Design review of the part built by this model. Coordinates are the model's own, in mm. Face numbers are marked on the shaded views. A direction names the side the tool comes from. Round coordinates to 2 decimals unless told otherwise and drop trailing zeros. Order: outer loops, then holes, each group sorted by start corner. A loop starts at its lowest first (then second) coordinate and runs counter-clockwise, first axis right, second up. Notation, with made-up numbers: M 56.25,-1.5 L 109.25,-1.5 A18 cw 109.25,25.5 Z; hole C 2,82.25 d10. An arc over 180 degrees is marked long. Use a Markdown table: item, result. Add a question column.
(1) Take a section at C-C (z = 0). Count the separate pieces of the cut face and the enclosed holes in it, then the cut area to 3 significant figures.
(2) For pin 1 (7 mm diameter, centred on y = 0, z = 0, fed in from +X); pin 2 (1.5 mm diameter, centred on x = -0.5, y = -9, fed in from -Z); pin 3 (2 mm diameter, centred on y = 8.5, z = 0, fed in from +X); pin 4 (3.5 mm diameter, centred on x = 0, z = 0, fed in from -Y), all flat-tipped, find the tip position at first contact; note any pin that passes through.
(3) Machinability: for the marked faces 1, 2 and 3, which of the approach directions +Z, -Z, +X, -X, +Y, -Y give a long, thin tool a straight path to every point of the face, cutting with its end or side? Answer none if there is none.
(4) The part is to be moulded in two halves that separate along Y. For the marked faces 4, 5 and 6, say which applies: released by +Y, released by -Y, zero draft, split by the parting line, or undercut.
(5) Take a section at A-A (x = 2.75). Write out the cut boundary in (y, z).
(6) To check wall thickness, follow probe 1 along Y at (x, z) = (0.25, 4); probe 2 along Y at (x, z) = (-6.75, 1); probe 3 along Y at (x, z) = (0, -1.5). State the ranges of each line that lie inside material, in increasing order. Write a range as from..to.
(7) Take a section at B-B (y = 0). Write out the cut boundary in (x, z).
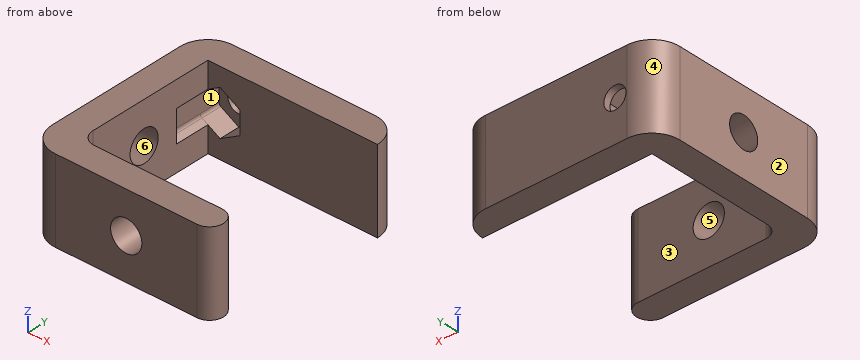
```python
from build123d import *

# Parameters (mm, degrees)
RESSALTO_EXTRUS_O1_DEPTH = 6
ESBO_O3_R                = 1.6
CORTE_EXTRUS_O1_DEPTH    = 4
CORTE_EXTRUS_O2_DEPTH    = 3
CORTE_EXTRUS_O3_DEPTH    = 5
FILETE1_R                = 0.5
FILETE2_R                = 4
FILETE3_R                = 2
ESBO_O6_R                = 2.25
CORTE_EXTRUS_O4_DEPTH    = 10
ESBO_O7_R                = 2.25
CORTE_EXTRUS_O5_DEPTH    = 10


# Some blends are built 0.0001 mm under size
with BuildPart() as part:
    # Esboço1 → Ressalto-extrusão1 (new, symmetric)
    with BuildSketch(Plane.XY):
        Polygon((14.2, 14.2), (-14.2, 14.2), (-14.2, -14.2), (14.2, -14.2), (14.2, -10.2), (10.2, -10.2), (-10.2, -10.2), (-10.2, 10.2), (10.2, 10.2), (14.2, 10.2), align=None)
    extrude(amount=RESSALTO_EXTRUS_O1_DEPTH, both=True)

    # Esboço3 → Corte-extrusão1 (cut)
    with BuildSketch(Plane(origin=(0, 14.2, 0), x_dir=(1, 0, 0), z_dir=(0, 1, 0))):
        with Locations(Location((-8.45, 0, 0), (0, 0, 270))):
            Circle(ESBO_O3_R)
    extrude(amount=-CORTE_EXTRUS_O1_DEPTH, mode=Mode.SUBTRACT)

    # Esboço4 → Corte-extrusão2 (cut)
    with BuildSketch(Plane.XZ.offset(-10.2)):
        Polygon((-8.45, 3.290896534), (-11.3, 1.645448267), (-11.3, -1.645448267), (-8.45, -3.290896534), (-5.6, -1.645448267), (-5.6, 1.645448267), align=None)
    extrude(amount=-CORTE_EXTRUS_O2_DEPTH, mode=Mode.SUBTRACT)

    # Esboço5 → Corte-extrusão3 (cut)
    with BuildSketch(Plane.XZ.offset(-10.2)):
        Polygon((-11.3, -1.645448267), (-10.2, -2.280533563), (-8.45, -3.290896534), (-5.6, -1.645448267), (-5.6, 1.645448267), (-8.45, 3.290896534), (-10.2, 2.280533563), (-11.3, 1.645448267), align=None)
    extrude(amount=CORTE_EXTRUS_O3_DEPTH, mode=Mode.SUBTRACT)

    # Filete1
    filete1_edges = [part.edges().sort_by_distance(p)[0] for p in [
        (-11.3, 9.2, -1.645448267),
        (-11.3, 9.2, 1.645448267),
        (-11.3, 5.2, 0),
    ]]
    fillet(filete1_edges, radius=FILETE1_R)

    # Filete2
    filete2_edges = [part.edges().sort_by_distance(p)[0] for p in [
        (-14.2, -14.2, 0),
        (-14.2, 14.2, 0),
        (14.2, 14.2, 0),
        (14.2, -14.2, 0),
    ]]
    fillet(filete2_edges, radius=FILETE2_R - 0.0001)  # a hair under: the kernel refuses the full size

    # Filete3
    # the kernel refuses this fillet: 2 mm, written as the material it adds along each edge
    with BuildSketch(Plane(origin=(-10.2, -10.2, -6), x_dir=(0, 1, 0), z_dir=(0, 0, 1))) as filete3_piece_1:
        with BuildLine():
            CenterArc((FILETE3_R, -FILETE3_R), FILETE3_R, 90, 90)
            Line((0, -FILETE3_R), (0, 0))
            Line((0, 0), (FILETE3_R, 0))
        make_face()
    extrude(amount=12)
    # the kernel refuses this fillet: 2 mm, written as the material it takes off along each edge
    with BuildSketch(Plane(origin=(14.2, -10.2, -20.141946005), x_dir=(-1, 0, 0), z_dir=(0, 0, 1))) as filete3_2_piece_1:
        with BuildLine():
            CenterArc((3.999896367, 2), FILETE3_R, 90.000104073, 179.999895927)
            Line((3.999892734, 4), (3.999892371, 4.2))
            ThreePointArc((3.999892371, 4.2), (-0.2, 0.0001), (-0.2, 0))
            Line((-0.2, 0), (0, -0.2))
            Line((0, -0.2), (3.999896367, -0.2))
            Line((3.999896367, -0.2), (3.999896367, 0))
        make_face()
    extrude(amount=40.283892009, mode=Mode.SUBTRACT)

    # Esboço6 → Corte-extrusão4 (cut)
    with BuildSketch(Plane.ZY.offset(14.2)):
        Circle(ESBO_O6_R)
    extrude(amount=-CORTE_EXTRUS_O4_DEPTH, mode=Mode.SUBTRACT)

    # Esboço7 → Corte-extrusão5 (cut)
    with BuildSketch(Plane.XZ.offset(14.2)):
        with Locations(Location((0, 0, 0), (0, 0, 270))):
            Circle(ESBO_O7_R)
    extrude(amount=-CORTE_EXTRUS_O5_DEPTH, mode=Mode.SUBTRACT)


solid = part.part
```
Verdict:
| question | item | result |
|---|---|---|
| 1 | separate pieces | 4 |
| 1 | enclosed holes | 0 |
| 1 | area | 228 mm^2 |
| 2 | pin 1 | stops at x = -10.2 |
| 2 | pin 2 | passes through |
| 2 | pin 3 | stops at x = -11.3 |
| 2 | pin 4 | stops at y = 10.2 |
| 3 | face 1 | none |
| 3 | face 2 | +Z, -Z, -X, +Y, -Y |
| 3 | face 3 | +Z, -Z, +X |
| 4 | face 4 | released by +Y |
| 4 | face 5 | zero draft |
| 4 | face 6 | undercut |
| 5 | outline | M -14.2,-6 L -10.2,-6 L -10.2,6 L -14.2,6 Z; M 10.2,-6 L 14.2,-6 L 14.2,6 L 10.2,6 Z |
| 6 | probe 1 | y = -14.2..-10.2, 10.2..14.2 |
| 6 | probe 2 | y = -14.2..-10.2, 13.2..14.2 |
| 6 | probe 3 | y = 10.2..14.2 |
| 7 | outline | M -14.2,-6 L -10.2,-6 L -10.2,-2.25 L -14.2,-2.25 Z; M -14.2,2.25 L -10.2,2.25 L -10.2,6 L -14.2,6 Z |
